Geometry: final body of the model. Coordinates: model frame, mm. A direction names the side the tool comes from. Round coordinates to 2 decimals unless told otherwise and drop trailing zeros. Order: outer loops, then holes, each group sorted by start corner. A loop starts at its lowest first (then second) coordinate and runs counter-clockwise, first axis right, second up. Notation, with made-up numbers: (56, 20) -> (62, 20) arc R23 ccw to (62, 59) -> close; hole circle Ø10 at (-18.75, 40). An arc over 180 degrees is marked (long way). Put each result on its own line as item: value.
```python
from build123d import *

# Parameters (mm, degrees)
F0_W     = 50.8
F0_H     = 44.45
F1_DEPTH = 31.75
F3_DEPTH = 76.2
F4_W     = 25.4
F4_H     = 19.05
F5_DEPTH = 25.4


with BuildPart() as f1:
    # F0 (on Front) → F1 (new body)
    with BuildSketch(Plane.XZ):
        with Locations((25.4, 22.225)):
            Rectangle(F0_W, F0_H)
    extrude(amount=F1_DEPTH)

    # F2 (on face) → F3 (cut)
    with BuildSketch(Plane.YZ.offset(50.8)):
        with BuildLine():
            Line((-31.75, 44.45), (-31.75, 12.7))
            ThreePointArc((-31.75, 12.7), (-13.444399, 24.090519), (-6.35, 44.45))
            Line((-6.35, 44.45), (-31.75, 44.45))
        make_face()
    extrude(amount=-F3_DEPTH, mode=Mode.SUBTRACT)

    # F4 (on face) → F5 (cut)
    with BuildSketch(Plane(origin=(0, 0, 0), x_dir=(-1, 0, 0), z_dir=(0, 1, 0))):
        with Locations((-25.4, 34.925)):
            Rectangle(F4_W, F4_H)
    extrude(amount=-F5_DEPTH, mode=Mode.SUBTRACT)


solid = f1.part
```
1. Cut plane C-C on y = -10.5. Return loops of the section in (x, z).
Ans:
outline: (0, 0) -> (50.8, 0) -> (50.8, 28.46) -> (38.1, 28.46) -> (38.1, 25.4) -> (12.7, 25.4) -> (12.7, 28.46) -> (0, 28.46) -> close
2. Draft query along X for faces 3 (the face through (26, -6, 25.4)), 4 (the face through (50.8, -12, 17)), 5 (the face through (25, -31.75, 6)). Return one class per face: +X half, -X half, draft (parallel to the pull), parting line (faces both ways), or undercut.
Ans:
face 3: undercut
face 4: +X half
face 5: draft
3. Cut plane B-B on x = 37. Return loops of the section in (y, z).
Ans:
outline: (-31.75, 0) -> (0, 0) -> (0, 25.4) -> (-12.45, 25.4) arc R32.38 cw to (-31.75, 12.7) -> close
4. Cut plane D-D on y = -7. Return loops of the section in (x, z), and give its area (3 significant figures).
Ans:
outline: (0, 0) -> (50.8, 0) -> (50.8, 37.86) -> (38.1, 37.86) -> (38.1, 25.4) -> (12.7, 25.4) -> (12.7, 37.86) -> (0, 37.86) -> close
area: 1,610 mm²
5. Contact query for flat-ended pins moving along their axis: P1, Ø5, axis at x = 16.5, z = 19.5, coming from the -Y side; P2, Ø3, axis at x = 27, z = 22.5, coming from the -Y side; P3, Ø4, axis at x = 35, y = -8, coming from the +Z side. Output: stop coordinate, or through.
Ans:
P1: y = -21.35
P2: y = -16.26
P3: z = 25.4
6. Cut plane A-A on z = 38. Return loops of the section in (x, y), and give its area (3 significant figures).
Ans:
outline: (0, -6.97) -> (12.7, -6.97) -> (12.7, 0) -> (0, 0) -> close; (38.1, -6.97) -> (50.8, -6.97) -> (50.8, 0) -> (38.1, 0) -> close
area: 177 mm²
7. Set-up query: faces 1 (the face through (0, -12, 17)), 2 (the face through (38.1, -5, 33)). Return all of +Z, -Z, +X, -X, +Y, -Y with unobstructed straight access to the full face (end or side cutting, diameter ignored); none if empty.
Ans:
face 1: +Z, -Z, -X, +Y, -Y
face 2: +Z, +Y, -Y
8. Material intervals for probe 1 along X at (y, z) = (-9, 30.5); probe 2 along Z at (x, y) = (23, -4.5); probe 3 along Z at (x, y) = (12.5, -29), sorted ascending.
Ans:
probe 1: 0 to 12.7, 38.1 to 50.8
probe 2: 0 to 25.4
probe 3: 0 to 13.43
